Read the model definition and answer for the solid it produces. Units are mm, in the model's axes. A direction names the side the tool comes from. Coordinates: 2 decimals unless noted, no trailing zeros. Write each loop counter-clockwise with the first axis right and the second up, starting at its lowest first coordinate (ties: lowest second). Pieces come first, ordered by that corner, then holes.
(1) Section C-C on x = -71.5 is taken. Write down the section's boundary in (y, z).
(2) Given pin 1 (1.6 mm diameter, centred on x = -77, y = 2.5, fed in from +Z); pin 2 (2 mm diameter, centred on y = 6, z = -73, fed in from +X); pin 3 (2 mm diameter, centred on x = -77.5, y = -1, fed in from +Z), each flat-ended and moving along its own axis, determine where each tip first touches the part or whether it passes through.
(3) Section B-B on y = 1.5 is taken. Write down the section's boundary in (x, z), then the cut area to 3 significant figures.
(4) Section A-A on y = -1 is taken. Write down the section's boundary in (x, z), then the cut area to 3 significant figures.
(5) Find the intervals of material crossed by probe 1 along X at (y, z) = (9, -70); probe 2 along X at (y, z) = (4, -70.25); probe 3 along Y at (x, z) = (-69.5, -72.25), in increasing order.
(6) Which of the six approach directions +Z, -Z, +X, -X, +Y, -Y give full straight-line access (tool end or side, diameter ignored) to faces 3 (the cylindrical face through (-58.63, 7.37, -66.83)), 4 (the flat face through (-77, -2, -66.371)), 5 (the flat face through (-77, 2, -69.371)), 6 (the flat face through (-77, -1, -75.154)), 7 (the flat face through (-57, 10, -70))?
(7) Section D-D on y = 8.25 is taken. Write down the section's boundary in (x, z).
(8) The mould has two halves that part along X. Classify faces 1 (the flat face through (-76.86, 0.51, -66.88)), 2 (the flat face through (-97, 10, -70)): +X half, -X half, draft (parallel to the pull), parting line (faces both ways), or undercut.
Autodesk Inventor part; units mm, degrees
ref_plane "YZ Plane" through (0, 0, 0) normal (1, 0, 0) x (0, 1, 0)
ref_plane "XZ Plane" through (0, 0, 0) normal (0, 1, 0) x (-1, 0, 0)
ref_plane "XY Plane" through (0, 0, 0) normal (0, 0, 1) x (1, 0, 0)
sketch "Skizze1" plane through (0, 0, 0) normal (0, 1, 0) x (-1, 0, 0)
  line L0 (96.8973, -70.154) -> (56.8973, -70.154)
  circle A0 centre (56.8973, -70.154) radius 5
  circle A1 centre (96.8973, -70.154) radius 5
  circle A2 centre (96.8973, -70.154) radius 3.75
  circle A3 centre (56.8973, -70.154) radius 3.75
  line L1 (96.8973, -65.154) -> (56.8973, -65.154)
  line L2 (56.8973, -65.154) -> (56.8973, -75.154)
  line L3 (56.8973, -75.154) -> (96.8973, -75.154)
  line L4 (96.8973, -75.154) -> (96.8973, -65.154)
  dimension "d8" = 10
  dimension "d11" = 10
  dimension "d12" = 7.5
  dimension "d15" = 7.5
  dimension "d18" = 40
extrude "Extrusion1" add sketch "Skizze1" along normal blind 10 contours A3 L2 L0 | L0 L2 A3 | L2 A3 | A2 L4 L0 | L0 L4 A2 | L4 A2
extrude "Extrusion2" add sketch "Skizze1" along normal blind 5 contours A0 L2 A3 L0 | L0 A3 L2 A0 | A1 L4 A2 L0 | L0 A2 L4 A1 | L2 A3 A0 | A1 L4 A2
extrude "Extrusion3" add sketch "Skizze1" along normal blind 3 and the other way blind 4.5 contours A0 L2 A3 L0 | A0 L1 A1 L0 | L0 A3 L2 A0 | L0 A1 L3 A0 | A3 L2 L0 | L0 L2 A3 | A1 L4 A2 L0 | L0 A2 L4 A1 | A2 L4 L0 | L0 L4 A2
fillet "Rundung1" radius 1 2 edges at (-51.8973, 5, -70.154) (-91.8973, 5, -70.154)
fillet "Rundung2" radius 0.2 2 edges at (-53.1473, 10, -70.154) (-93.1473, 10, -70.154)
extrude "Extrusion4" add sketch "Skizze1" against normal blind 4.5 contours A0 L2 A3 L0 | L0 A3 L2 A0 | A3 L2 L0 | L0 L2 A3 | A1 L4 A2 L0 | L0 A2 L4 A1 | L2 A3 A0 | L2 A3 | A2 L4 L0 | L0 L4 A2 | A1 L4 A2 | L4 A2
sketch "Skizze2" plane through (0, -4.5, 0) normal (0, -1, 0) x (1, 0, 0)
  line L0 (-96.8973, -65.154) -> (-56.8973, -65.154)
  line L1 (-74.3973, -65.154) -> (-79.3973, -65.154)
  line L2 (-79.3973, -65.154) -> (-79.3973, -66.3709)
  line L3 (-79.3973, -66.3709) -> (-74.3973, -66.3709)
  line L4 (-74.3973, -66.3709) -> (-74.3973, -65.154)
  point P0 (0, 0)
  dimension "d31" = 5
  dimension "d32" = 17.5
extrude "Extrusion5" cut sketch "Skizze2" against normal blind 10
sketch "Skizze3" plane through (0, 3, 0) normal (0, 1, 0) x (1, 0, 0)
  line L0 (-74.3973, 66.3709) -> (-79.3973, 66.3709)
  line L1 (-74.3973, 66.3709) -> (-79.3973, 66.3709)
  line L2 (-79.3973, 66.3709) -> (-79.3973, 69.3709)
  line L3 (-79.3973, 69.3709) -> (-74.3973, 69.3709)
  line L4 (-74.3973, 69.3709) -> (-74.3973, 66.3709)
  point P0 (0, 0)
  dimension "d35" = 3
extrude "Extrusion6" cut sketch "Skizze3" against normal blind 2
chamfer "Fase1" distance 1 angle 45 1 edges at (-76.8973, 1, -66.3709)
properties part number "2er-Stecker"
Response:
1. outline: (-4.5, -75.15) - (3, -75.15) - (3, -65.15) - (-4.5, -65.15) - close
2. pin 1: stops at z = -69.37
2. pin 2: stops at x = -53.63
2. pin 3: stops at z = -66.37
3. outline: (-96.9, -75.15) - (-56.9, -75.15) arc R5 ccw to (-56.9, -65.15) - (-74.4, -65.15) - (-74.4, -69.37) - (-79.4, -69.37) - (-79.4, -65.15) - (-96.9, -65.15) arc R5 ccw to start
3. area: 457 mm2
4. outline: (-96.9, -75.15) - (-56.9, -75.15) arc R5 ccw to (-56.9, -65.15) - (-74.4, -65.15) - (-74.4, -66.37) - (-79.4, -66.37) - (-79.4, -65.15) - (-96.9, -65.15) arc R5 ccw to start
4. area: 472 mm2
5. probe 1: x = -100.64 to -93.15, -60.64 to -53.15
5. probe 2: x = -101.9 to -91.9, -61.9 to -51.9
5. probe 3: y = -4.5 to 3
6. face 3: +Y
6. face 4: +Z, +Y, -Y
6. face 5: +Z, +Y
6. face 6: -Z, +X, -X, +Y, -Y
6. face 7: +Z, -Z, +X, -X, +Y
7. outline: circle Ø7.5 at (-96.9, -70.15); circle Ø7.5 at (-56.9, -70.15)
8. face 1: undercut
8. face 2: draft
